Can you work these out from the model? Positions are in its coordinate system, mm. A direction names the side the tool comes from. Coordinates: 2 decimals unless noted, no trailing zeros. Loops run counter-clockwise (first coordinate to the right, second up) from the corner with the lowest first, then second, coordinate; pieces in that order, holes last.
```python
from build123d import *

# Parameters (mm, degrees)
SKETCH4_R               = 2.375
BOSS_EXTRUDE2_DEPTH     = 1.5
SKETCH5_OUTSIDE_W       = 64.264
SKETCH5_OUTSIDE_H       = 63.182
SKETCH5_OUTSIDE_R       = 3.5
CUT_EXTRUDE1_DEPTH      = 15
CUT_EXTRUDE1_DRAFT      = -60
MIRROR1_COPY_1_SKETCH_W = 64.264
MIRROR1_COPY_1_SKETCH_H = 63.182
MIRROR1_COPY_1_SKETCH_R = 3.5
MIRROR1_COPY_1_DEPTH    = 15
MIRROR1_COPY_1_DRAFT    = -60
SKETCH4_3_R             = 2.375
BOSS_EXTRUDE3_DEPTH     = 15
FILLET1_R               = 1
FILLET2_R               = 0.5


with BuildPart() as part:
    # Sketch4 → Boss-Extrude2 (new, symmetric)
    with BuildSketch(Plane.XY):
        Polygon((4.041451884, 0), (2.020725942, 3.5), (-2.020725942, 3.5), (-4.041451884, 0), (-2.020725942, -3.5), (2.020725942, -3.5), align=None)
        Circle(SKETCH4_R, mode=Mode.SUBTRACT)
        Circle(SKETCH4_R)
    extrude(amount=BOSS_EXTRUDE2_DEPTH, both=True)


with BuildPart() as cut_extrude1_tool:
    # Sketch5 outside → Cut-Extrude1 (with draft: the straight prism first)
    with BuildSketch(Plane.XY.offset(1.5)):
        Rectangle(SKETCH5_OUTSIDE_W, SKETCH5_OUTSIDE_H)
        Circle(SKETCH5_OUTSIDE_R, mode=Mode.SUBTRACT)
    extrude(amount=-CUT_EXTRUDE1_DEPTH)
    # Cut-Extrude1: the draft: its side faces are tilted about the plane it starts from
    cut_extrude1_sides = [cut_extrude1_tool.faces().sort_by_distance(p)[0] for p in [
        (0, -31.591, -6),
        (32.132, 0, -6),
        (0, 31.591, -6),
        (-32.132, 0, -6),
        (-3.5, 0, -6),
    ]]
    draft(cut_extrude1_sides, Plane.XY.offset(1.5), CUT_EXTRUDE1_DRAFT)


with BuildPart() as part_1:
    add(part.part)

    # Cut-Extrude1: cut by cut_extrude1_tool
    add(cut_extrude1_tool.part, mode=Mode.SUBTRACT)


with BuildPart() as mirror1_copy_1_tool:
    # Mirror1 copy 1 sketch → Mirror1 copy 1 (with draft: the straight prism first)
    with BuildSketch(Plane(origin=(0, 0, -1.5), x_dir=(1, 0, 0), z_dir=(0, 0, -1))):
        Rectangle(MIRROR1_COPY_1_SKETCH_W, MIRROR1_COPY_1_SKETCH_H)
        Circle(MIRROR1_COPY_1_SKETCH_R, mode=Mode.SUBTRACT)
    extrude(amount=-MIRROR1_COPY_1_DEPTH)
    # Mirror1 copy 1: the draft: its side faces are tilted about the plane it starts from
    mirror1_copy_1_sides = [mirror1_copy_1_tool.faces().sort_by_distance(p)[0] for p in [
        (0, -31.591, 6),
        (32.132, 0, 6),
        (0, 31.591, 6),
        (-32.132, 0, 6),
        (-3.5, 0, 6),
    ]]
    draft(mirror1_copy_1_sides, Plane(origin=(0, 0, -1.5), x_dir=(1, 0, 0), z_dir=(0, 0, -1)), MIRROR1_COPY_1_DRAFT)


with BuildPart() as part_2:
    add(part_1.part)

    # Mirror1 copy 1: cut by mirror1_copy_1_tool
    add(mirror1_copy_1_tool.part, mode=Mode.SUBTRACT)

    # Sketch4_3 → Boss-Extrude3 (add)
    with BuildSketch(Plane.XY):
        Circle(SKETCH4_3_R)
    extrude(amount=BOSS_EXTRUDE3_DEPTH)

    # Fillet1
    fillet1_edges = [part_2.edges().sort_by_distance(p)[0] for p in [
        (4.041451884, 0, 0),
        (2.020725942, -3.5, 0),
        (-2.020725942, -3.5, 0),
        (-4.041451884, 0, 0),
        (-2.020725942, 3.5, 0),
        (2.020725942, 3.5, 0),
    ]]
    fillet(fillet1_edges, radius=FILLET1_R)

    # Fillet2
    fillet2_edges = [part_2.edges().sort_by_distance(p)[0] for p in [
        (-2.375, 0, 15),
    ]]
    fillet(fillet2_edges, radius=FILLET2_R)


solid = part_2.part
```
Item 1: Suppose I cut it at C-C, the plane z = 4.5. Please give me the cut outline in (x, y) (3 decimals).
Results are:
outline: circle Ø4.75 at (0, 0)
Item 2: I need wall thicknesses on line 1 along X through (y, z) = (0.5, 1); line 2 along Z through (x, y) = (3.25, 0.75); line 3 along Y through (x, z) = (-2, 7.5). Which ranges of each line are inside material? Lowest first, please.
Results are:
line 1: x = -3.75 to 3.75
line 2: z = -1.5 to 1.5
line 3: y = -1.28 to 1.28
Item 3: On a 3-axis mill with a long thin cutter (end or side, diameter ignored), from which of +Z, -Z, +X, -X, +Y, -Y can I reach the whole of each face in a straight line? I mean faces 1 (the face through (1.096, -2.107, 7.909)), 2 (the face through (1.95, 3.36, 0.02)). Say none if no direction works.
Results are:
face 1: +Z
face 2: +Z, -Z, +X, +Y
Item 4: I'm going to push flat-ended pins straight in: P1, Ø1, axis at x = -2, z = 10.5, coming from the +Y side; P2, Ø1.5, axis at x = -2.5, y = 1.5, coming from the +Z side. Where does each tip first touch, or does it pass through?
Results are:
P1: stops at y = 1.84
P2: stops at z = 14.91
Item 5: Suppose I cut it at A-A, the plane z = 0.5. Please give me the cut outline in (x, y), plus the area to 3 significant figures.
Results are:
outline: (-3.75, -0.5) - (-2.31, -3) arc R1 ccw to (-1.44, -3.5) - (1.44, -3.5) arc R1 ccw to (2.31, -3) - (3.75, -0.5) arc R1 ccw to (3.75, 0.5) - (2.31, 3) arc R1 ccw to (1.44, 3.5) - (-1.44, 3.5) arc R1 ccw to (-2.31, 3) - (-3.75, 0.5) arc R1 ccw to start
area: 42.1 mm2
Item 6: Suppose I cut it at B-B, the plane y = 0. Please give me the cut outline in (x, z) (3 decimals).
Results are:
outline: (-3.887, -1.277) - (-3.5, -1.5) - (3.5, -1.5) - (3.887, -1.277) - (3.887, 1.277) - (3.5, 1.5) - (2.375, 1.5) - (2.375, 14.5) arc R0.5 ccw to (1.875, 15) - (-1.875, 15) arc R0.5 ccw to (-2.375, 14.5) - (-2.375, 1.5) - (-3.5, 1.5) - (-3.887, 1.277) - close
